```python
from build123d import *

# Parameters (mm, degrees)
SKETCH1_W           = 20
SKETCH1_H           = 3
SKETCH1_W_2         = 3
SKETCH1_H_2         = 20
SKETCH1_W_3         = 5
SKETCH1_H_3         = 50
BOSS_EXTRUDE1_DEPTH = 3


with BuildPart() as part:
    # Sketch1 → Boss-Extrude1 (new body)
    with BuildSketch(Plane.XY):
        with BuildLine():
            Line((10, -62), (10, -65))
            Line((10, -65), (35, -65))
            Line((35, -65), (35, -63.5))
            ThreePointArc((35, -63.5), (36.65, -61.85), (38.3, -63.5))
            Line((38.3, -63.5), (38.3, -65))
            Line((38.3, -65), (65, -65))
            Line((65, -65), (65, -33.3))
            Line((65, -33.3), (63.5, -33.3))
            ThreePointArc((63.5, -33.3), (61.85, -31.65), (63.5, -30))
            Line((63.5, -30), (65, -30))
            Line((65, -30), (65, -10))
            Line((65, -10), (62, -10))
            Line((62, -10), (62, 10))
            Line((62, 10), (65, 10))
            Line((65, 10), (65, 30))
            Line((65, 30), (63.5, 30))
            ThreePointArc((63.5, 30), (61.85, 31.65), (63.5, 33.3))
            Line((63.5, 33.3), (65, 33.3))
            Line((65, 33.3), (65, 65))
            Line((65, 65), (38.3, 65))
            Line((38.3, 65), (38.3, 63.5))
            ThreePointArc((38.3, 63.5), (36.65, 61.85), (35, 63.5))
            Line((35, 63.5), (35, 65))
            Line((35, 65), (10, 65))
            Line((10, 65), (10, 62))
            Line((10, 62), (-10, 62))
            Line((-10, 62), (-10, 65))
            Line((-10, 65), (-35, 65))
            Line((-35, 65), (-35, 63.5))
            ThreePointArc((-35, 63.5), (-36.65, 61.85), (-38.3, 63.5))
            Line((-38.3, 63.5), (-38.3, 65))
            Line((-38.3, 65), (-65, 65))
            Line((-65, 65), (-65, 33.3))
            Line((-65, 33.3), (-63.5, 33.3))
            ThreePointArc((-63.5, 33.3), (-61.85, 31.65), (-63.5, 30))
            Line((-63.5, 30), (-65, 30))
            Line((-65, 30), (-65, 10))
            Line((-65, 10), (-62, 10))
            Line((-62, 10), (-62, -10))
            Line((-62, -10), (-65, -10))
            Line((-65, -10), (-65, -30))
            Line((-65, -30), (-63.5, -30))
            ThreePointArc((-63.5, -30), (-61.85, -31.65), (-63.5, -33.3))
            Line((-63.5, -33.3), (-65, -33.3))
            Line((-65, -33.3), (-65, -65))
            Line((-65, -65), (-38.3, -65))
            Line((-38.3, -65), (-38.3, -63.5))
            ThreePointArc((-38.3, -63.5), (-36.65, -61.85), (-35, -63.5))
            Line((-35, -63.5), (-35, -65))
            Line((-35, -65), (-10, -65))
            Line((-10, -65), (-10, -62))
            Line((-10, -62), (10, -62))
        make_face()
        with Locations((-40.5, -57.5)):
            Rectangle(SKETCH1_W, SKETCH1_H, mode=Mode.SUBTRACT)
        with Locations((-59.5, -35)):
            Rectangle(SKETCH1_W_2, SKETCH1_H_2, mode=Mode.SUBTRACT)
        with Locations((-5.5, -57.5)):
            Rectangle(SKETCH1_W, SKETCH1_H, mode=Mode.SUBTRACT)
        with Locations((13.5, -35)):
            Rectangle(SKETCH1_W_2, SKETCH1_H_2, mode=Mode.SUBTRACT)
        with Locations((57.5, -35)):
            Rectangle(SKETCH1_W_3, SKETCH1_H_3, mode=Mode.SUBTRACT)
        with Locations((-59.5, 0)):
            Rectangle(SKETCH1_W_2, SKETCH1_H_2, mode=Mode.SUBTRACT)
        with Locations((-59.5, 35)):
            Rectangle(SKETCH1_W_2, SKETCH1_H_2, mode=Mode.SUBTRACT)
        with Locations((-40.5, 57.5)):
            Rectangle(SKETCH1_W, SKETCH1_H, mode=Mode.SUBTRACT)
        with Locations((-5.5, 57.5)):
            Rectangle(SKETCH1_W, SKETCH1_H, mode=Mode.SUBTRACT)
        with Locations((13.5, 0)):
            Rectangle(SKETCH1_W_2, SKETCH1_H_2, mode=Mode.SUBTRACT)
        with BuildLine():
            ThreePointArc((38, 31), (43, 36), (48, 31))
            Line((48, 31), (48, 21))
            ThreePointArc((48, 21), (43, 16), (38, 21))
            Line((38, 21), (38, 31))
        make_face(mode=Mode.SUBTRACT)
        with Locations((13.5, 35)):
            Rectangle(SKETCH1_W_2, SKETCH1_H_2, mode=Mode.SUBTRACT)
    extrude(amount=BOSS_EXTRUDE1_DEPTH)


solid = part.part
```
The model under review builds one solid part; all positions refer to its coordinate system, in mm. A direction names the side the tool comes from. Round coordinates to 2 decimals unless told otherwise and drop trailing zeros. Order: outer loops, then holes, each group sorted by start corner. A loop starts at its lowest first (then second) coordinate and runs counter-clockwise, first axis right, second up. Notation, with made-up numbers: (31.5, 76) -> (40.5, 76) arc R8 ccw to (40.5, 81) -> close; hole circle Ø4 at (61, 70.5). An arc over 180 degrees is marked (long way). One line per item, written item: value. Start each with the question number.
Q1. Take a section at D-D (z = 0.65). Count the separate pieces of the cut face and the enclosed holes in it, and give its area (3 significant figures).
Q2. Wall thickness on line 1 (Y direction, x = -47.5, z = 1.75); line 2 (X direction, y = -4.5, z = 0.8); line 3 (Y direction, x = -2, z = 0.4): over which ranges is each line inside the solid? List them lowest first.
Q3. Take a section at A-A (y = -37). Write out the cut boundary in (x, z), and give its area (3 significant figures).
Q4. Machinability: for faces 4 (the face through (-10, 63, 1)), 5 (the face through (36.61, -61.85, 1.48)), 6 (the face through (43, 16, 1)), which of the approach directions +Z, -Z, +X, -X, +Y, -Y give a long, thin tool a straight path to every point of the face, cutting with its end or side? Answer none if there is none.
Q5. Take a section at C-C (x = -1). Write out the cut boundary in (y, z), and give its area (3 significant figures).
Q6. Mouldability with a two-part tool opening along X and no side actions: class faces 1 (the face through (61.85, -31.69, 1.48)), 2 (the face through (51, -65, 1)), 3 (the face through (-6, -59, 1)) as released by +X, released by -X, zero draft, split by the parting line, or undercut.
Q7. Take a section at B-B (x = 13.5). Write out the cut boundary in (y, z), and give its area (3 significant figures).
Reported:
1. separate pieces: 1
1. enclosed holes: 12
1. area: 15,600 mm2
2. line 1: y = -65 to -59, -56 to 56, 59 to 65
2. line 2: x = -62 to -61, -58 to 12, 15 to 62
2. line 3: y = -62 to -59, -56 to 56, 59 to 62
3. outline: (-65, 0) -> (-61, 0) -> (-61, 3) -> (-65, 3) -> close; (-58, 0) -> (12, 0) -> (12, 3) -> (-58, 3) -> close; (15, 0) -> (55, 0) -> (55, 3) -> (15, 3) -> close; (60, 0) -> (65, 0) -> (65, 3) -> (60, 3) -> close
3. area: 357 mm2
4. face 4: +Z, -Z, +Y
4. face 5: +Z, -Z, -Y
4. face 6: +Z, -Z
5. outline: (-62, 0) -> (-59, 0) -> (-59, 3) -> (-62, 3) -> close; (-56, 0) -> (56, 0) -> (56, 3) -> (-56, 3) -> close; (59, 0) -> (62, 0) -> (62, 3) -> (59, 3) -> close
5. area: 354 mm2
6. face 1: released by +X
6. face 2: zero draft
6. face 3: undercut
7. outline: (-65, 0) -> (-45, 0) -> (-45, 3) -> (-65, 3) -> close; (-25, 0) -> (-10, 0) -> (-10, 3) -> (-25, 3) -> close; (10, 0) -> (25, 0) -> (25, 3) -> (10, 3) -> close; (45, 0) -> (65, 0) -> (65, 3) -> (45, 3) -> close
7. area: 210 mm2
